Can you work these out from the model? Positions are in its coordinate system, mm. A direction names the side the tool comes from. Give positions to 0.01 mm unless a question says otherwise; leave off trailing zeros. Order: outer loops, then holes, each group sorted by start corner. A loop starts at its lowest first (then second) coordinate and runs counter-clockwise, first axis right, second up. Notation, with made-up numbers: (57, -33) - (84, -33) arc R12 ccw to (84, -24) - close; hole circle Ø1 at (-39.75, 79). An arc over 180 degrees is marked (long way). Use one line per item in the form item = value. Start each with the question number.
1) Suppose I cut it at B-B, the plane x = 76.5. Write out the boundary of the cut face in (y, z) (3 decimals).
2) We'd pull the mould along X, two halves only. Please class faces 4 (the cylindrical face through (-41.61, 6.26, 14.3)), 5 (the cylindrical face through (64.91, -17.05, 14.3)), 6 (the flat face through (58, 14, -2)): released by +X, released by -X, zero draft, split by the parting line, or undercut.
3) For pin 1 (14 mm diameter, centred on x = 58.5, z = -7, fed in from -Y); pin 2 (3 mm diameter, centred on y = -15, z = 7, fed in from +X); pin 3 (6.5 mm diameter, centred on x = 56.5, z = 4, fed in from +Y); pin 4 (13.5 mm diameter, centred on y = 0, z = 0, fed in from +X), each with a flat end and sliding along its axis, tell me the tip position at first contact or that it passes through.
4) Please list where these lines run through material, in increasing order: probe 1 along Y at (x, z) = (52, 12); probe 2 along Z at (x, y) = (-59.5, 0); probe 3 along Y at (x, z) = (-42, 12).
5) Suppose I cut it at D-D, the plane y = -9. Write out the boundary of the cut face in (x, z) (3 decimals).
6) Suppose I cut it at C-C, the plane z = 3. Write out the boundary of the cut face in (x, y).
7) Which directions (+Z, -Z, +X, -X, +Y, -Y) give clear straight access to the entire face, cutting with the end or side of a thin tool? Please do faces 1 (the flat face through (74, -18, 14)), 2 (the flat face through (44, -26, 14)), 3 (the flat face through (44, 26, 14)).
8) Suppose I cut it at A-A, the plane y = -26. Write out the boundary of the cut face in (x, z) (3 decimals), and give its area (3 significant figures).
```python
from build123d import *

# Parameters (mm, degrees)
SKETCH1_W                  = 32
SKETCH1_H                  = 28
SKETCH1_R                  = 7.5692
BOSS_EXTRUDE1_DEPTH        = 64
SKETCH5_W                  = 102.6
SKETCH5_H                  = 28
CUT_EXTRUDE1_DEPTH         = 9.475
CUT_EXTRUDE1_DEPTH_BACK    = 33.147
F_10_CLEARANCE_HOLE1_D     = 5.6134
F_10_CLEARANCE_HOLE1_DEPTH = 25.4
F_10_CLEARANCE_HOLE1_TIP   = 1.686435499
BOSS_EXTRUDE2_DEPTH        = 9.525
F_10_CLEARANCE_HOLE2_D     = 5.6134
FILLET2_R                  = 3.175


with BuildPart() as part:
    # Sketch1 → Boss-Extrude1 (new body, symmetric)
    with BuildSketch(Plane(origin=(0, 0, 0), x_dir=(0, 0, -1), z_dir=(1, 0, 0))):
        with Locations((-3, 0)):
            Rectangle(SKETCH1_W, SKETCH1_H)
        Circle(SKETCH1_R, mode=Mode.SUBTRACT)
    extrude(amount=BOSS_EXTRUDE1_DEPTH, both=True)

    # Sketch5 → Cut-Extrude1 (cut, two sides)
    with BuildSketch(Plane.XY) as cut_extrude1_sk:
        Rectangle(SKETCH5_W, SKETCH5_H)
    extrude(amount=CUT_EXTRUDE1_DEPTH, mode=Mode.SUBTRACT)
    extrude(cut_extrude1_sk.sketch, amount=-CUT_EXTRUDE1_DEPTH_BACK, mode=Mode.SUBTRACT)

    # #10 Clearance Hole1
    with Locations(Plane(origin=(-39.55789498, -3.670822781, 9.475), x_dir=(-1, 0, 0), z_dir=(0, 0, -1))):
        with Locations((1.44210502, -5.329177219), (1.44210502, 12.670822781)):
            Hole(F_10_CLEARANCE_HOLE1_D / 2, depth=F_10_CLEARANCE_HOLE1_DEPTH)
            with Locations((0, 0, -(F_10_CLEARANCE_HOLE1_DEPTH + F_10_CLEARANCE_HOLE1_TIP / 2))):  # 118° drill point
                Cone(0, F_10_CLEARANCE_HOLE1_D / 2, F_10_CLEARANCE_HOLE1_TIP, mode=Mode.SUBTRACT)

    # Sketch7 → Boss-Extrude2 (add)
    with BuildSketch(Plane(origin=(0, 0, 9.475), x_dir=(-1, 0, 0), z_dir=(0, 0, -1))):
        Polygon((-44, -14), (-64, -14), (-64, -18), (-82, -18), (-82, -34), (-44, -34), align=None)
    boss_extrude2 = extrude(amount=-BOSS_EXTRUDE2_DEPTH)

    # #10 Clearance Hole2 (through all)
    with Locations(Plane(origin=(0, 0, 9.475), x_dir=(-1, 0, 0), z_dir=(0, 0, -1))):
        with Locations((-76.5, -26), (-52, -26)):
            f_10_clearance_hole2 = Hole(F_10_CLEARANCE_HOLE2_D / 2)

    # Mirror2: Boss-Extrude2, #10 Clearance Hole2 across plane
    add(boss_extrude2.mirror(Plane.ZX))
    add(f_10_clearance_hole2.mirror(Plane.ZX), mode=Mode.SUBTRACT)

    # Fillet2
    fillet2_edges = [part.edges().sort_by_distance(p)[0] for p in [
        (44, 14, 14.2375),
        (44, -14, 14.2375),
        (64, 18, 14.2375),
        (64, -18, 14.2375),
    ]]
    fillet(fillet2_edges, radius=FILLET2_R)


solid = part.part
```
Result sheet:
q1.outline = (-34, 9.475) - (-28.807, 9.475) - (-28.807, 19) - (-34, 19) - close; (-23.193, 9.475) - (-18, 9.475) - (-18, 19) - (-23.193, 19) - close; (18, 9.475) - (23.193, 9.475) - (23.193, 19) - (18, 19) - close; (28.807, 9.475) - (34, 9.475) - (34, 19) - (28.807, 19) - close
q2.face_4 = undercut
q2.face_5 = released by +X
q2.face_6 = zero draft
q3.pin_1 = -14
q3.pin_2 = 64
q3.pin_3 = 14
q3.pin_4 = through
q4.probe_1 = -34 to -28.81, -23.19 to 23.19, 28.81 to 34
q4.probe_2 = -13 to -7.57, 7.57 to 19
q4.probe_3 = -14 to -11.62, -6.38 to 6.38, 11.62 to 14
q5.outline = (-64, -13) - (-51.3, -13) - (-51.3, 9.475) - (-43.807, 9.475) - (-43.807, 19) - (-64, 19) - close; (-38.193, 9.475) - (51.3, 9.475) - (51.3, -13) - (64, -13) - (64, 19) - (-38.193, 19) - close
q6.outline = (-64, -14) - (-51.3, -14) - (-51.3, -6.95) - (-64, -6.95) - close; (-64, 6.95) - (-51.3, 6.95) - (-51.3, 14) - (-64, 14) - close; (51.3, -14) - (64, -14) - (64, -6.95) - (51.3, -6.95) - close; (51.3, 6.95) - (64, 6.95) - (64, 14) - (51.3, 14) - close
q7.face_1 = +Z, -Z, +X
q7.face_2 = +Z, -Z, -X, -Y
q7.face_3 = +Z, -Z, -X, +Y
q8.outline = (44, 9.475) - (49.193, 9.475) - (49.193, 19) - (44, 19) - close; (54.807, 9.475) - (73.693, 9.475) - (73.693, 19) - (54.807, 19) - close; (79.307, 9.475) - (82, 9.475) - (82, 19) - (79.307, 19) - close
q8.area = 255 mm²
